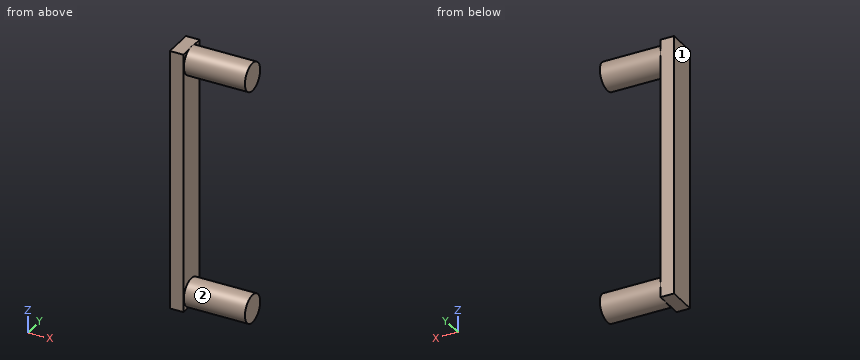
```python
from build123d import *

# Parameters (mm, degrees)
F0_W     = 15.5
F0_H     = 34
F1_DEPTH = 300
F2_R     = 16
F3_DEPTH = 70


with BuildPart() as f1:
    # F0 (on Top) → F1 (new body)
    with BuildSketch(Plane.XY):
        with Locations((7.75, -17)):
            Rectangle(F0_W, F0_H)
    extrude(amount=F1_DEPTH)

    # F2 (on face) → F3 (join)
    with BuildSketch(Plane.YZ.offset(15.5)):
        with Locations((-17, 285)):
            Circle(F2_R)
        with Locations((-17, 15)):
            Circle(F2_R)
    extrude(amount=F3_DEPTH)


solid = f1.part
```
Geometry: final body of the model. Coordinates: model frame, mm. Face numbers are marked on the shaded views. Round coordinates to 2 decimals unless told otherwise and drop trailing zeros. Order: outer loops, then holes, each group sorted by start corner. A loop starts at its lowest first (then second) coordinate and runs counter-clockwise, first axis right, second up. Notation, with made-up numbers: M 23,53 L 33,53 A17 cw 33,57 Z; hole C 75,-21 d3. An arc over 180 degrees is marked long. One line per item, written item: value.
(1) Pin query (flat end, axial travel): P1, Ø5, axis at y = -27.5, z = 123.5, coming from the +X side; P2, Ø4.5, axis at x = 10.5, y = -17.5, coming from the +Z side; P3, Ø8, axis at x = 7, y = -9.5, coming from the -Z side. Return the tip coordinate at first contact, or that it passes through.
Result sheet:
P1: x = 15.5
P2: z = 300
P3: z = 0
(2) Cut plane C-C (x = 63.5). Return the cut outline in (y, z), and give its area (3 significant figures).
Result sheet:
outline: C -17,15 d32; C -17,285 d32
area: 1,610 mm2
(3) Cut plane A-A (z = 15). Return the cut outline in (x, y).
Result sheet:
outline: M 0,-34 L 15.5,-34 L 15.5,-33 L 85.5,-33 L 85.5,-1 L 15.5,-1 L 15.5,0 L 0,0 Z
(4) Line query: probe 1 along Z at (x, y) = (77, -18); probe 2 along X at (y, z) = (-8, 114); probe 3 along Z at (x, y) = (9, -18.5). Output: solid intervals per line, ascending. Write a range as [from, to].
Result sheet:
probe 1: [-0.97, 30.97], [269.03, 300.97]
probe 2: [0, 15.5]
probe 3: [0, 300]
(5) Pull-direction query (Z, two-part tool) for the marked faces 1 and 2; classes: pulls with the +Z half, pulls with the -Z half, needs draft (parallel to the pull), parting line crosses it, or undercut.
Result sheet:
face 1: needs draft
face 2: undercut
(6) Cut plane D-D (z = 274). Return the cut outline in (x, y), and give its area (3 significant figures).
Result sheet:
outline: M 0,-34 L 15.5,-34 L 15.5,-28.62 L 85.5,-28.62 L 85.5,-5.38 L 15.5,-5.38 L 15.5,0 L 0,0 Z
area: 2,150 mm2
(7) Cut plane B-B (y = -17). Return the cut outline in (x, z), and give its area (3 significant figures).
Result sheet:
outline: M 0,0 L 15.5,0 L 15.5,-1 L 85.5,-1 L 85.5,31 L 15.5,31 L 15.5,269 L 85.5,269 L 85.5,301 L 15.5,301 L 15.5,300 L 0,300 Z
area: 9,130 mm2
